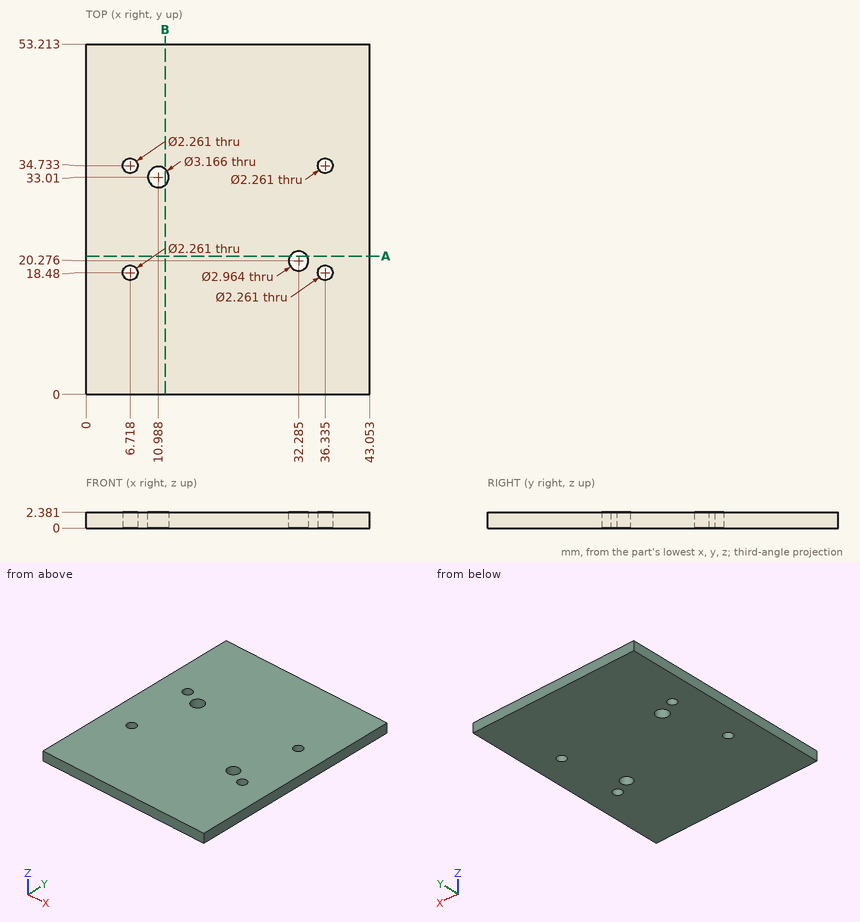
Drawing for the job (mm, zero at the part's lowest x, y, z). Give positions to 0.01 mm unless a question says otherwise; leave off trailing zeros. Loops run counter-clockwise (first coordinate to the right, second up) from the corner with the lowest first, then second, coordinate; pieces in that order, holes last.
1) Drop a flat-ended pin along its axis: P1, Ø2, axis at x = 6.72, y = 18.48, coming from the -Z side. Give the stop position or say it passes through.
Values follow:
P1: passes through
2) Probe line 1 along Y through (x, z) = (33, 1.1) (1 decimal); line 2 along Y through (x, z) = (7, 0.2) (1 decimal); line 3 along Y through (x, z) = (10.5, 2.3) (1 decimal). List the from-to ranges inside material, lowest first.
Values follow:
line 1: y = 0 to 19, 21.6 to 53.2
line 2: y = 0 to 17.4, 19.6 to 33.6, 35.8 to 53.2
line 3: y = 0 to 31.5, 34.5 to 53.2
3) Band-saw the part on B-B on x = 12. List the corners of the cut face in (y, z).
Values follow:
outline: (0, 0) - (31.79, 0) - (31.79, 2.38) - (0, 2.38) - close; (34.23, 0) - (53.21, 0) - (53.21, 2.38) - (34.23, 2.38) - close
4) Band-saw the part on A-A on y = 21. List the corners of the cut face in (x, z).
Values follow:
outline: (0, 0) - (30.99, 0) - (30.99, 2.38) - (0, 2.38) - close; (33.58, 0) - (43.05, 0) - (43.05, 2.38) - (33.58, 2.38) - close
